```python
from build123d import *

# Parameters (mm, degrees)
SALIENTE_EXTRUIR1_DEPTH = 10
CROQUIS2_R              = 20
CORTAR_EXTRUIR1_DEPTH   = 10
CROQUIS3_R              = 20
CORTAR_EXTRUIR2_DEPTH   = 10
CROQUIS5_W              = 60
CROQUIS5_H              = 10
SALIENTE_EXTRUIR3_DEPTH = 55
SALIENTE_EXTRUIR4_DEPTH = 9
CROQUIS8_R              = 20
CORTAR_EXTRUIR3_DEPTH   = 9
CROQUIS9_R              = 20
CORTAR_EXTRUIR4_DEPTH   = 10


with BuildPart() as part:
    # Croquis1 → Saliente-Extruir1 (new body)
    with BuildSketch(Plane(origin=(0, 0, 0), x_dir=(1, 0, 0), z_dir=(0, 1, 0))):
        with BuildLine():
            Line((0, 26.904276051), (128.079511341, 26.904276051))
            ThreePointArc((128.079511341, 26.904276051), (154.983787391, 0), (128.079511341, -26.904276051))
            Line((128.079511341, -26.904276051), (0, -26.904276051))
            ThreePointArc((0, -26.904276051), (-26.904276051, 0), (0, 26.904276051))
        make_face()
    extrude(amount=SALIENTE_EXTRUIR1_DEPTH)

    # Croquis2 → Cortar-Extruir1 (cut)
    with BuildSketch(Plane.XZ):
        with Locations(Location((0, 0, 0), (0, 0, 270))):
            Circle(CROQUIS2_R)
    extrude(amount=-CORTAR_EXTRUIR1_DEPTH, mode=Mode.SUBTRACT)

    # Croquis3 → Cortar-Extruir2 (cut)
    with BuildSketch(Plane(origin=(0, 10, 0), x_dir=(1, 0, 0), z_dir=(0, 1, 0))):
        with Locations(Location((127.980340476, 0, 0), (0, 0, 270))):
            Circle(CROQUIS3_R)
    extrude(amount=-CORTAR_EXTRUIR2_DEPTH, mode=Mode.SUBTRACT)

    # Croquis5 → Saliente-Extruir3 (add)
    with BuildSketch(Plane(origin=(0, 0, 0), x_dir=(-1, 0, 0), z_dir=(0, -1, 0))):
        with Locations((-58.558456053, -21.904276051)):
            Rectangle(CROQUIS5_W, CROQUIS5_H)
        with Locations((-58.558456053, 21.904276051)):
            Rectangle(CROQUIS5_W, CROQUIS5_H)
    extrude(amount=SALIENTE_EXTRUIR3_DEPTH)

    # Croquis7 → Saliente-Extruir4 (add)
    with BuildSketch(Plane(origin=(0, -55, 0), x_dir=(-1, 0, 0), z_dir=(0, -1, 0))):
        with BuildLine():
            Line((0, -26.950667307), (-127.980340476, -26.950667307))
            ThreePointArc((-127.980340476, -26.950667307), (-154.931007783, 0), (-127.980340476, 26.950667307))
            Line((-127.980340476, 26.950667307), (0, 26.950667307))
            ThreePointArc((0, 26.950667307), (26.950667307, 0), (0, -26.950667307))
        make_face()
    extrude(amount=SALIENTE_EXTRUIR4_DEPTH)

    # Croquis8 → Cortar-Extruir3 (cut)
    with BuildSketch(Plane(origin=(0, -64, 0), x_dir=(-1, 0, 0), z_dir=(0, -1, 0))):
        with Locations(Location((-129.139989333, 0, 0), (0, 0, 90))):
            Circle(CROQUIS8_R)
    extrude(amount=-CORTAR_EXTRUIR3_DEPTH, mode=Mode.SUBTRACT)

    # Croquis9 → Cortar-Extruir4 (cut)
    with BuildSketch(Plane(origin=(0, -64, 0), x_dir=(-1, 0, 0), z_dir=(0, -1, 0))):
        with Locations(Location((0, 0, 0), (0, 0, 90))):
            Circle(CROQUIS9_R)
    extrude(amount=-CORTAR_EXTRUIR4_DEPTH, mode=Mode.SUBTRACT)


solid = part.part
```
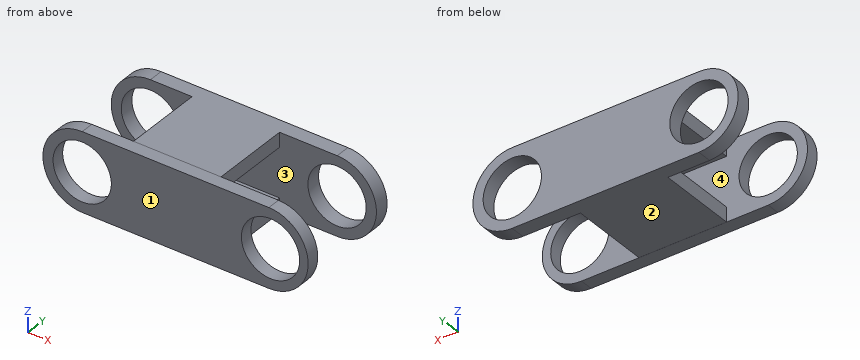
Could you check a few things on this model? Use its own coordinates, in mm. Face numbers are marked on the shaded views. Round coordinates to 2 decimals unless told otherwise and drop trailing zeros. Loops run counter-clockwise (first coordinate to the right, second up) from the corner with the lowest first, then second, coordinate; pieces in that order, holes last. Notation, with made-up numbers: M 19.5,71.5 L 53.5,71.5 A7 cw 53.5,81.5 Z; hole C 56.25,-30.5 d1. An arc over 180 degrees is marked long. Answer as CSV lines item,"result".
1) For pin 1 Ø1.5 at (x, y) = (54, -46.5) entering from -Z; pin 2 Ø12 at (x, y) = (34.5, -11.5) entering from +Z; pin 3 Ø2 at (x, y) = (26, -15) entering from -Z; pin 4 Ø8 at (y, z) = (-29.5, -21) entering from -X, each with a flat end and sliding along its axis, tell me the tip position at first contact or that it passes through.
From the geometry:
pin 1,"z = -26.9"
pin 2,"z = 26.9"
pin 3,"through"
pin 4,"x = 28.56"
2) If I drill on probe 1 along X at (y, z) = (4.25, 0); probe 2 along X at (y, z) = (-58, 0); probe 3 along Y at (x, z) = (146, 19.5), over which ranges is the centre line in solid material (lowest first)?
From the geometry:
probe 1,"-26.9 to -20, 20 to 107.98, 147.98 to 154.98"
probe 2,"-26.95 to -20, 20 to 109.14, 149.14 to 154.93"
probe 3,"-64 to -55, 0 to 10"
3) We'd pull the mould along Y, two halves only. Please class the marked faces 1, 2, 3 and 4: released by +Y, released by -Y, zero draft, split by the parting line, or undercut.
From the geometry:
face 1,"released by -Y"
face 2,"zero draft"
face 3,"undercut"
face 4,"undercut"
4) Imagine slicing it at D-D on z = -11. List the corners of the cut face in (x, y) for me.
From the geometry:
outline,"M -24.6,-64 L -16.7,-64 L -16.7,-55 L -24.6,-55 Z; M -24.55,0 L -16.7,0 L -16.7,10 L -24.55,10 Z; M 16.7,-64 L 112.44,-64 L 112.44,-55 L 16.7,-55 Z; M 16.7,0 L 111.28,0 L 111.28,10 L 16.7,10 Z; M 144.68,0 L 152.63,0 L 152.63,10 L 144.68,10 Z; M 145.84,-64 L 152.58,-64 L 152.58,-55 L 145.84,-55 Z"
5) Imagine slicing it at C-C on x = 105. List the corners of the cut face in (y, z) for me.
From the geometry:
outline,"M -64,-26.95 L -55,-26.95 L -55,26.95 L -64,26.95 Z; M 0,-26.9 L 10,-26.9 L 10,26.9 L 0,26.9 Z"
6) Imagine slicing it at A-A on y = -14. List the corners of the cut face in (x, z) for me.
From the geometry:
outline,"M 28.56,-26.9 L 88.56,-26.9 L 88.56,-16.9 L 28.56,-16.9 Z; M 28.56,16.9 L 88.56,16.9 L 88.56,26.9 L 28.56,26.9 Z"
7) Imagine slicing it at B-B on z = 0. List the corners of the cut face in (x, y) for me, and give its area (3 significant figures).
From the geometry:
outline,"M -26.95,-64 L -20,-64 L -20,-55 L -26.95,-55 Z; M -26.9,0 L -20,0 L -20,10 L -26.9,10 Z; M 20,-64 L 109.14,-64 L 109.14,-55 L 20,-55 Z; M 20,0 L 107.98,0 L 107.98,10 L 20,10 Z; M 147.98,0 L 154.98,0 L 154.98,10 L 147.98,10 Z; M 149.14,-64 L 154.93,-64 L 154.93,-55 L 149.14,-55 Z"
area,"1,940 mm^2"
